Build history of the part. All positions in model axes, mm. A direction names the side the tool comes from. Round coordinates to 2 decimals unless told otherwise and drop trailing zeros. Write each loop counter-clockwise with the first axis right and the second up, starting at its lowest first coordinate (ties: lowest second). Pieces come first, ordered by that corner, then holes. Notation, with made-up numbers: (16.5, 70) -> (70.5, 70) arc R28 cw to (70.5, 107) -> close; hole circle Ø9 at (74, 18). An arc over 180 degrees is marked (long way). One line per question, with ' | ' between items.
from build123d import *

# Parameters (mm, degrees)
EXTRUDE_1_DEPTH             = 1500
CUT_EXTRUDE_874_DEPTH       = 1510.610877014
SKETCH_4_R                  = 6.6
CUT_EXTRUDE_1154_DEPTH      = 1510.387292911
CUT_EXTRUDE_3058_DEPTH      = 1510.610877014
CUT_EXTRUDE_3058_DEPTH_BACK = 1510.610877014
CUT_EXTRUDE_6_DEPTH         = 1534.297101021
CUT_EXTRUDE_6_DEPTH_BACK    = 1534.297101021
SKETCH_19_R                 = 4
PATTERN_LINEAR_1_COUNT      = 9
PATTERN_LINEAR_1_PITCH      = 145
PATTERN_LINEAR_2_COUNT      = 10
PATTERN_LINEAR_2_PITCH      = 150


with BuildPart() as part:
    # Эскиз1 → Бобышка-Вытянуть1 (new body)
    with BuildSketch(Plane.XY):
        with BuildLine():
            Line((70, -155), (8, -155))
            ThreePointArc((8, -155), (2.343145751, -152.656854249), (0, -147))
            Line((0, -147), (0, 147))
            ThreePointArc((0, 147), (2.343145751, 152.656854249), (8, 155))
            Line((8, 155), (70, 155))
            Line((70, 155), (70, 150))
            Line((70, 150), (8, 150))
            ThreePointArc((8, 150), (5.878679656, 149.121320344), (5, 147))
            Line((5, 147), (5, -147))
            ThreePointArc((5, -147), (5.878679656, -149.121320344), (8, -150))
            Line((8, -150), (70, -150))
            Line((70, -150), (70, -155))
        make_face()
    extrude(amount=EXTRUDE_1_DEPTH)

    # Эскиз2 → Cut-Extrude 874 (cut, through all)
    with BuildSketch(Plane.ZY):
        Polygon((1500, 155), (1416.935750346, -155), (1500, -155), align=None)
    extrude(amount=-CUT_EXTRUDE_874_DEPTH, mode=Mode.SUBTRACT)

    # Эскиз4 → Cut-Extrude 1154 (cut, through all)
    with BuildSketch(Plane(origin=(5, 0, 0), x_dir=(0, 0, -1), z_dir=(1, 0, 0))):
        with Locations(Location((-1292.5, 0, 0), (0, 0, 90))):
            Circle(SKETCH_4_R)
        with Locations(Location((-1273.75, 32.475952642, 0), (0, 0, 90))):
            Circle(SKETCH_4_R)
        with Locations(Location((-1273.75, -32.475952642, 0), (0, 0, 90))):
            Circle(SKETCH_4_R)
    extrude(amount=-CUT_EXTRUDE_1154_DEPTH, mode=Mode.SUBTRACT)

    # Эскиз7 → Зенковка для винта с потайной головкой и внутренним шестигранником M61 (revolve, cut)
    with BuildSketch(Plane(origin=(40, -155, 1229.935750346), x_dir=(0, 0, -1), z_dir=(1, 0, 0))):
        Polygon((0, 0), (0, 31.982840043), (3.3, 30), (3.3, 3.555), (6.855, 0), align=None)
    hole_wizard_m61 = revolve(axis=Axis((40, -161.35, 1229.935750346), (0, 1, 0)), mode=Mode.SUBTRACT)

    # Эскиз16 → Cut-Extrude 3058 (cut, two sides: drawn at the far end of the back side and taken through both)
    with BuildSketch(Plane.ZY.offset(-CUT_EXTRUDE_3058_DEPTH_BACK)):
        Polygon((1434.702880481, 89.617739901), (1408.717448353, -7.361213059), (1412.967521989, -8.500016857), (1438.952954117, 88.478936102), align=None)
    extrude(amount=CUT_EXTRUDE_3058_DEPTH + CUT_EXTRUDE_3058_DEPTH_BACK, mode=Mode.SUBTRACT)

    # Эскиз19 → Вырез-Вытянуть6 (cut, two sides: drawn at the far end of the back side and taken through both)
    with BuildSketch(Plane(origin=(0, 155, 0), x_dir=(1, 0, 0), z_dir=(0, 1, 0)).offset(-CUT_EXTRUDE_6_DEPTH_BACK)):
        with Locations(Location((40, -1205, 0), (0, 0, 270))):
            Circle(SKETCH_19_R)
        with Locations(Location((40, -1105, 0), (0, 0, 270))):
            Circle(SKETCH_19_R)
    extrude(amount=CUT_EXTRUDE_6_DEPTH + CUT_EXTRUDE_6_DEPTH_BACK, mode=Mode.SUBTRACT)

    # Линейный массив1: Зенковка для винта с потайной головкой и внутренним шестигранником M61 ×9
    with Locations(*[(0, 0, -i * PATTERN_LINEAR_1_PITCH) for i in range(1, PATTERN_LINEAR_1_COUNT)]):
        add(hole_wizard_m61, mode=Mode.SUBTRACT)

    # Эскиз26 → Отверстие обработанное метчиком M82 (revolve, cut)
    with BuildSketch(Plane(origin=(45, 155, 1370), x_dir=(0, 0, 1), z_dir=(1, 0, 0))):
        Polygon((0, 0), (0, 24.292926105), (3.4, 22.25), (3.4, 0), align=None)
    hole_wizard_m82 = revolve(axis=Axis((45, 161.35, 1370), (0, -1, 0)), mode=Mode.SUBTRACT)

    # Линейный массив2: Отверстие обработанное метчиком M82 ×10
    with Locations(*[(0, 0, -i * PATTERN_LINEAR_2_PITCH) for i in range(1, PATTERN_LINEAR_2_COUNT)]):
        add(hole_wizard_m82, mode=Mode.SUBTRACT)


solid = part.part
(1) Mould opens along Y. For faces 4 (the flat face through (5, 2, 738)), 5 (the flat face through (39, 150, 739)), 6 (the flat face through (0, -2, 738)), 7 (the flat face through (39, -155, 699)) say: pulls with the +Y half, pulls with the -Y half, needs draft (parallel to the pull), parting line crosses it, or undercut.
Calculated:
face 4: undercut | face 5: undercut | face 6: needs draft | face 7: pulls with the -Y half
(2) Drop flat-ended pins along their axis: pin 1 (10 mm diameter, centred on y = 13, z = 863, fed in from +X); pin 2 (5.5 mm diameter, centred on x = 45, z = 320, fed in from +Y); pin 3 (11 mm diameter, centred on x = 45, z = 470, fed in from +Y); pin 4 (10.5 mm diameter, centred on x = 40, z = 69.94, fed in from -Y). Give the stop position or say it passes through.
Calculated:
pin 1: x = 5 | pin 2: y = -150 | pin 3: y = 155 | pin 4: y = -153.4
(3) 3-axis set-ups, long thin cutter, end or side, ignore diameter. For faces 1 (the flat face through (3.73, 0.72, 1458.66)), 2 (the flat face through (2.54, 39.31, 1425.78)), 3 (the flat face through (39, -150, 699)): which of +Z, -Z, +X, -X, +Y, -Y reach the whole face in a straight line?
Calculated:
face 1: +Z, +X, -X, -Y | face 2: +X, -X | face 3: +Z, -Z, +X
(4) Slice it at A-A (z = 1333.5). Write the cut outline in (x, y), then the cut area to 3 significant figures.
Calculated:
outline: (0, -147) arc R8 ccw to (8, -155) -> (70, -155) -> (70, -150) -> (8, -150) arc R3 cw to (5, -147) -> (5, 147) arc R3 cw to (8, 150) -> (70, 150) -> (70, 155) -> (8, 155) arc R8 ccw to (0, 147) -> close | area: 2,180 mm2
(5) Wall check: line 1 (Y direction, x = 29, z = 689); line 2 (X direction, y = -58, z = 978.5); line 3 (Y direction, x = 7, z = 1258). Give the ranges that are in metal, low to high. Write a range as from..to.
Calculated:
line 1: -155..-150, 150..155 | line 2: 0..5 | line 3: -154.94..-149.83, 149.83..154.94
(6) Slice it at B-B (y = -56). Write the cut outline in (x, z).
Calculated:
outline: (0, 0) -> (5, 0) -> (5, 1443.46) -> (0, 1443.46) -> close
